Can you work these out from the drawing? Everything is in mm from the part's minimum corner. A direction names the side the tool comes from. Round coordinates to 2 decimals unless told otherwise and drop trailing zeros. Order: outer loops, then holes, each group sorted by start corner. A loop starts at its lowest first (then second) coordinate and runs counter-clockwise, first axis right, second up. Notation, with made-up numbers: (27.5, -23) - (62.5, -23) arc R3 cw to (62.5, -18) - close; hole circle Ø7 at (14.5, 70). An arc over 180 degrees is marked (long way). Write item = value, one per line.
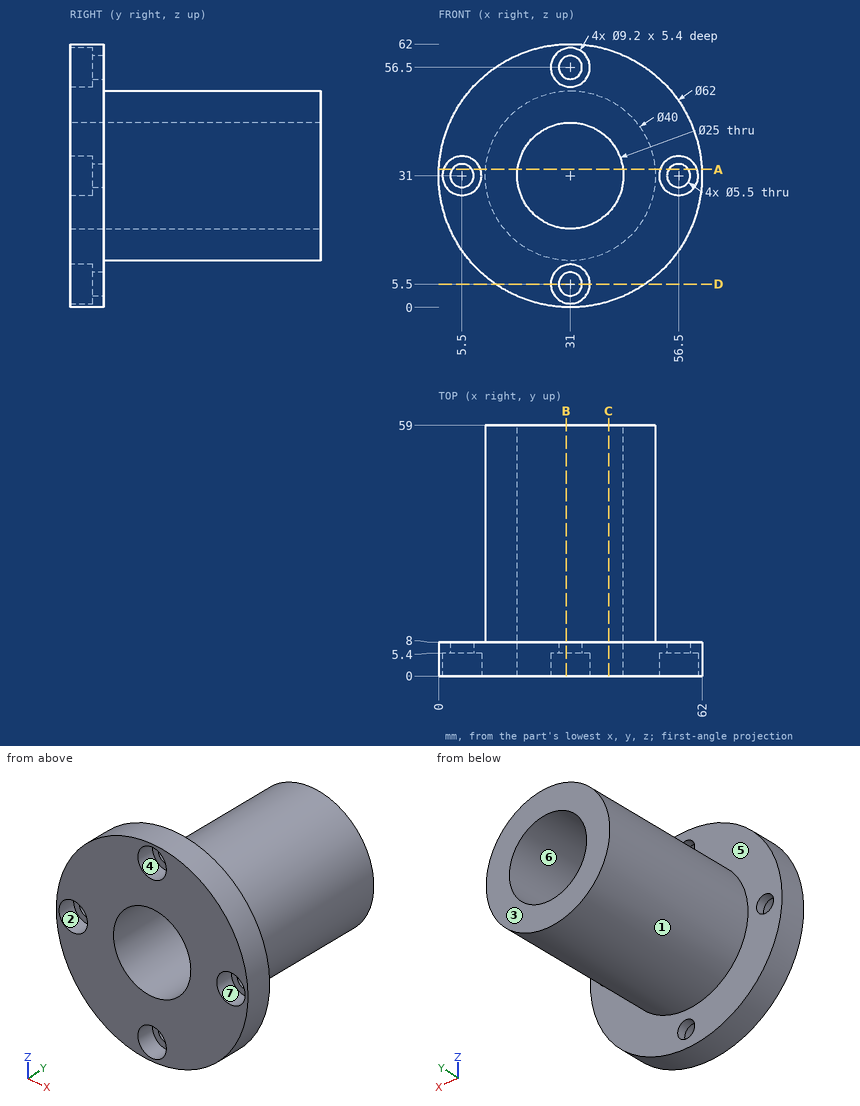
(1) If we section it at D-D (z = 5.5): Write out the boundary of the cut face in (x, y).
Computed:
outline = (13.37, 0) - (26.4, 0) - (26.4, 5.4) - (28.25, 5.4) - (28.25, 8) - (13.37, 8) - close; (33.75, 5.4) - (35.6, 5.4) - (35.6, 0) - (48.63, 0) - (48.63, 8) - (33.75, 8) - close
(2) If I drill on line 1 (X direction, y = 6.3, z = 31); line 2 (X direction, y = 1, z = 31); line 3 (Y direction, x = 54.5, z = 29), over which ranges is the centre line in solid material (lowest first)? Write a range as from..to.
Computed:
line_1 = 0..2.75, 8.25..18.5, 43.5..53.75, 59.25..62
line_2 = 0..0.9, 10.1..18.5, 43.5..51.9, 61.1..62
line_3 = 5.4..8
(3) Thinking about a two-plate mould opening in X: for the marked faces 1, 2, 3 and 4, which applies, +X half, -X half, draft (parallel to the pull), parting line (faces both ways), or undercut?
Computed:
face_1 = parting line
face_2 = undercut
face_3 = draft
face_4 = undercut
(4) If we section it at C-C (x = 40): Write out the boundary of the cut face in (y, z), plus the area to 3 significant figures.
Computed:
outline = (0, 1.34) - (8, 1.34) - (8, 13.14) - (59, 13.14) - (59, 22.33) - (0, 22.33) - close; (0, 39.67) - (59, 39.67) - (59, 48.86) - (8, 48.86) - (8, 60.66) - (0, 60.66) - close
area = 1,270 mm^2
(5) On a 3-axis mill with a long thin cutter (end or side, diameter ignored), from which of +Z, -Z, +X, -X, +Y, -Y can I reach the whole of each face in a straight line? I mean the marked faces 5, 6 and 7. Say none if no direction works.
Computed:
face_5 = +Y
face_6 = +Y, -Y
face_7 = -Y
(6) If we section it at B-B (x = 30): Write out the boundary of the cut face in (y, z), plus the area to 3 significant figures.
Computed:
outline = (0, 0.02) - (8, 0.02) - (8, 2.94) - (5.4, 2.94) - (5.4, 1.01) - (0, 1.01) - close; (0, 9.99) - (5.4, 9.99) - (5.4, 8.06) - (8, 8.06) - (8, 11.03) - (59, 11.03) - (59, 18.54) - (0, 18.54) - close; (0, 43.46) - (59, 43.46) - (59, 50.97) - (8, 50.97) - (8, 53.94) - (5.4, 53.94) - (5.4, 52.01) - (0, 52.01) - close; (0, 60.99) - (5.4, 60.99) - (5.4, 59.06) - (8, 59.06) - (8, 61.98) - (0, 61.98) - close
area = 939 mm^2
(7) Will these pins go through, and if not, where does the flat tip stop? P1, Ø4.5, axis at x = 29.5, z = 58, coming from the -Y side; P2, Ø1, axis at y = 44.5, z = 43, coming from the +X side; P3, Ø7, axis at x = 56.5, z = 31, coming from the +Y side.
Computed:
P1 = 5.4
P2 = 47.36
P3 = 8
(8) If we section it at A-A (z = 32.5): Write out the boundary of the cut face in (x, y), plus the area to 3 significant figures.
Computed:
outline = (0.04, 0) - (1.15, 0) - (1.15, 5.4) - (3.2, 5.4) - (3.2, 8) - (0.04, 8) - close; (7.8, 5.4) - (9.85, 5.4) - (9.85, 0) - (18.59, 0) - (18.59, 59) - (11.06, 59) - (11.06, 8) - (7.8, 8) - close; (43.41, 0) - (52.15, 0) - (52.15, 5.4) - (54.2, 5.4) - (54.2, 8) - (50.94, 8) - (50.94, 59) - (43.41, 59) - close; (58.8, 5.4) - (60.85, 5.4) - (60.85, 0) - (61.96, 0) - (61.96, 8) - (58.8, 8) - close
area = 947 mm^2
